Model file for the job. Use its own axes, mm. Face numbers are marked on the shaded views. Give positions to 0.01 mm unless a question says otherwise; leave off trailing zeros. Loops run counter-clockwise (first coordinate to the right, second up) from the corner with the lowest first, then second, coordinate; pieces in that order, holes last. Notation, with made-up numbers: M 87.25,39 L 98.25,39 A25 ccw 98.25,77 Z; hole C -3.5,50 d10. An arc over 180 degrees is marked long. Answer in a Markdown table with one row per item.
```python
from build123d import *

# Parameters (mm, degrees)
F0_R     = 79.7122
F1_DEPTH = 72.39
F2_R     = 25.4
F3_T     = -2.54


with BuildPart() as f1:
    # F0 (on Top) → F1 (new body)
    with BuildSketch(Plane.XY):
        with Locations((-31.042261, 11.334619)):
            Circle(F0_R)
    extrude(amount=F1_DEPTH)

    # F2
    f2_edges = [f1.edges().sort_by_distance(p)[0] for p in [
        (-110.754461, 11.334619, 72.39),
    ]]
    fillet(f2_edges, radius=F2_R)

    # F3
    f3_openings = [f1.faces().sort_by_distance(p)[0] for p in [
        (-31.042261, 11.334619, 0),
    ]]
    offset(amount=F3_T, openings=f3_openings)


solid = f1.part
```
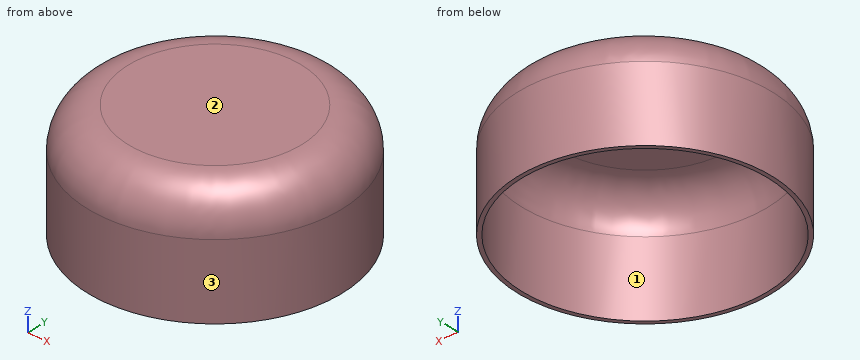
Q1. Drop flat-ended pins along their axis: pin 1 (6 mm diameter, centred on x = -5, z = 58.5, fed in from +Y); pin 2 (1.5 mm diameter, centred on y = 42, z = 57, fed in from -X); pin 3 (12 mm diameter, centred on y = -3.5, z = 16.5, fed in from +X). Give the stop position or say it passes through.
Reported:
| item | result |
|---|---|
| pin 1 | y = 85.5 |
| pin 2 | x = -102.85 |
| pin 3 | x = 48.18 |
Q2. Mould opens along X. For the marked faces 1, 2 and 3 say: released by +X, released by -X, zero draft, split by the parting line, or undercut.
Reported:
| item | result |
|---|---|
| face 1 | undercut |
| face 2 | zero draft |
| face 3 | split by the parting line |
Q3. Probe probe 1 along X at (y, z) = (13, 40); probe 2 along Y at (x, z) = (-31.5, 15.5); probe 3 along Y at (x, z) = (-79.5, 24.5). List the from-to ranges inside material, lowest first.
Reported:
| item | result |
|---|---|
| probe 1 | -110.74 to -108.2, 46.11 to 48.65 |
| probe 2 | -68.38 to -65.84, 88.51 to 91.05 |
| probe 3 | -51.96 to -48.73, 71.4 to 74.63 |
Q4. Saw through at A-A (z = 67). Give the cut face in (x, y), and give its area (3 significant figures).
Reported:
| item | result |
|---|---|
| outline | C -31.04,11.33 d139.91; hole C -31.04,11.33 d130.73 |
| area | 1,950 mm² |
Q5. Saw through at B-B (z = 51). Give the cut face in (x, y), and give its area (3 significant figures).
Reported:
| item | result |
|---|---|
| outline | C -31.04,11.33 d158.79; hole C -31.04,11.33 d153.64 |
| area | 1,260 mm² |
